Study the drawing (mm; zero at the part's minimum x, y, z) and answer. Give positions to 0.01 mm unless a question says otherwise; leave off trailing zeros. Order: outer loops, then holes, each group sorted by start corner. A loop starts at its lowest first (then second) coordinate and runs counter-clockwise, first axis right, second up.
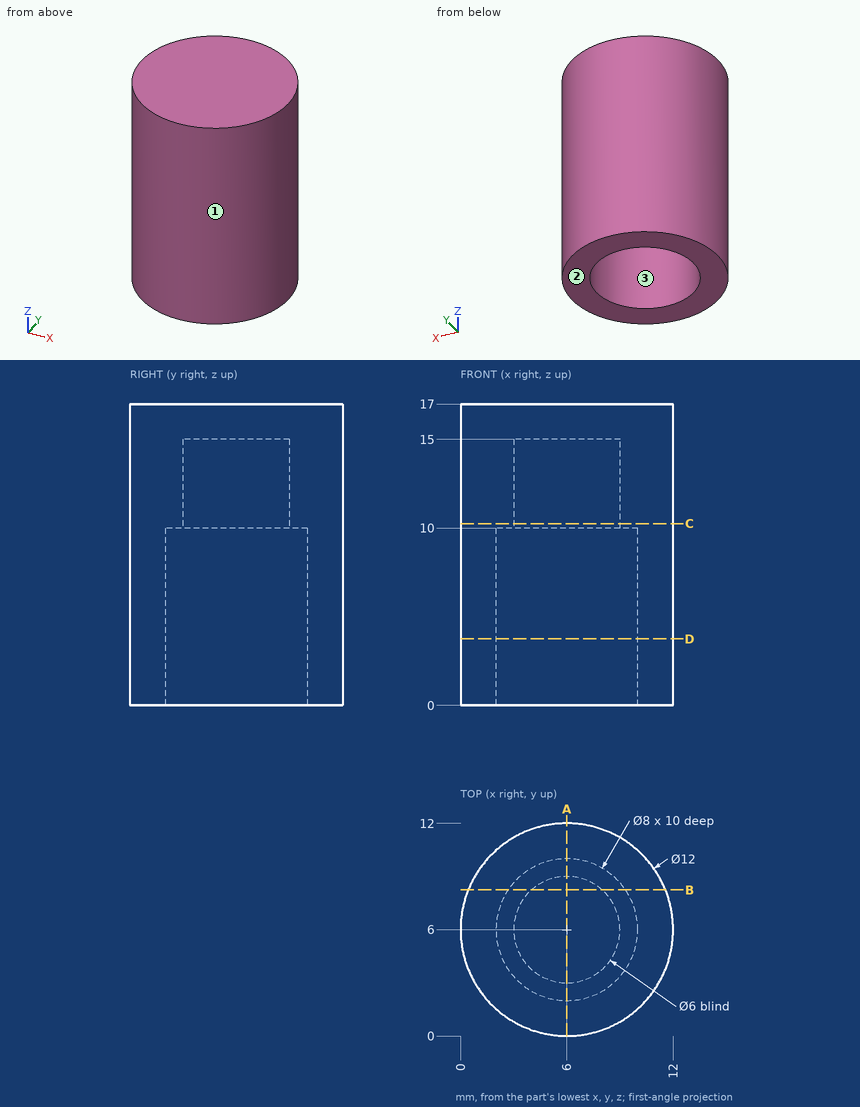
1) For a pull along X with two mould halves and no side action, classify the marked faces 1, 2 and 3 as +X half, -X half, draft (parallel to the pull), parting line (faces both ways), or undercut.
Geometry says:
face 1: parting line
face 2: draft
face 3: undercut
2) Find section B-B (y = 8.25). Write down the section's boundary in (x, z), then the cut area to 3 significant figures.
Geometry says:
outline: (0.44, 0) - (2.69, 0) - (2.69, 10) - (4.02, 10) - (4.02, 15) - (7.98, 15) - (7.98, 10) - (9.31, 10) - (9.31, 0) - (11.56, 0) - (11.56, 17) - (0.44, 17) - close
area: 103 mm2
3) Straight lines are drawn through the part: probe 1 along Y at (x, z) = (6, 13.85); probe 2 along Y at (x, z) = (6, 3.5); probe 3 along X at (y, z) = (8.25, 8.25). For each, find the intervals that lie inside material, in ascending order.
Geometry says:
probe 1: y = 0 to 3, 9 to 12
probe 2: y = 0 to 2, 10 to 12
probe 3: x = 0.44 to 2.69, 9.31 to 11.56
4) Given P1, Ø1.8, axis at x = 5, y = 6, coming from the -Z side; P2, Ø3, axis at x = 2.5, z = 7.5, coming from the -Y side; P3, Ø3, axis at y = 4, z = 6, coming from the +X side, each flat-ended and moving along its own axis, determine where each tip first touches the part or whether it passes through.
Geometry says:
P1: stops at z = 15
P2: stops at y = 0.34
P3: stops at x = 11.98
5) Find section C-C (z = 10.25). Write down the section's boundary in (x, y).
Geometry says:
outline: circle Ø12 at (6, 6); hole circle Ø6 at (6, 6)
6) Find section D-D (z = 3.75). Write down the section's boundary in (x, y).
Geometry says:
outline: circle Ø12 at (6, 6); hole circle Ø8 at (6, 6)
7) Find section A-A (x = 6). Write down the section's boundary in (y, z), then the cut area to 3 significant figures.
Geometry says:
outline: (0, 0) - (2, 0) - (2, 10) - (3, 10) - (3, 15) - (9, 15) - (9, 10) - (10, 10) - (10, 0) - (12, 0) - (12, 17) - (0, 17) - close
area: 94.0 mm2
